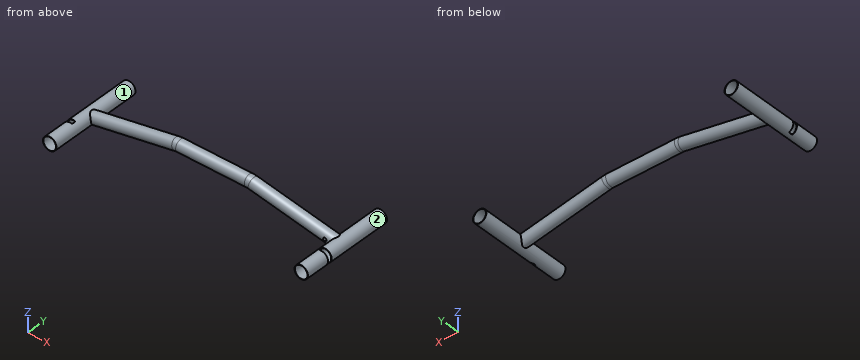
```python
from build123d import *

# Parameters (mm, degrees)
SKETCH2_R               = 11.1
SKETCH2_R_2             = 10.3
SKETCH3_R               = 12.7
SKETCH3_R_2             = 11.9
BOSS_EXTRUDE1_DEPTH     = 88
SKETCH4_R               = 11.9
CUT_EXTRUDE1_DEPTH      = 310.344523999
SKETCH5_R               = 10.7
CUT_EXTRUDE2_DEPTH      = 88
CUT_EXTRUDE3_DEPTH      = 20
CUT_EXTRUDE4_REACH      = 271.188
CUT_EXTRUDE4_END_RADIUS = 11.1
SKETCH8_R               = 3


with BuildPart() as part:
    # Sweep1: sweep along a path in Sketch1
    with BuildLine(Plane(origin=(0, 0, 0), x_dir=(1, 0, 0), z_dir=(0, 1, 0))) as sweep1_path:
        Line((232, 30), (72.22502534, 0.657923176))
        ThreePointArc((72.22502534, 0.657923176), (68.627459651, 0.164820366), (65, 0))
        Line((65, 0), (-65, 0))
        ThreePointArc((-65, 0), (-68.627459651, 0.164820366), (-72.22502534, 0.657923176))
        Line((-72.22502534, 0.657923176), (-232, 30))
    # Sketch2 → Sweep1 (sweep)
    with BuildSketch(Plane(origin=(232, 0, -30), x_dir=(-0.18062563349676417, 0, -0.9835519206040384), z_dir=(0.9835519206040384, 0, -0.18062563349676417))):
        Circle(SKETCH2_R)
        Circle(SKETCH2_R_2, mode=Mode.SUBTRACT)
    sweep(path=sweep1_path.line)

    # Sketch3 → Boss-Extrude1 (add, symmetric)
    with BuildSketch(Plane(origin=(0, 0, 0), x_dir=(1, 0, 0), z_dir=(0, 1, 0))):
        with Locations(Location((237.901311524, 31.083753801, 0), (0, 0, 270))):
            Circle(SKETCH3_R)
        with Locations(Location((237.901311524, 31.083753801, 0), (0, 0, 270))):
            Circle(SKETCH3_R_2, mode=Mode.SUBTRACT)
    boss_extrude1 = extrude(amount=BOSS_EXTRUDE1_DEPTH, both=True)

    # Sketch4 → Cut-Extrude1 (cut, through all)
    with BuildSketch(Plane.XZ.offset(88)):
        with Locations(Location((237.901311524, -31.083753801, 0), (0, 0, 90))):
            Circle(SKETCH4_R)
    cut_extrude1 = extrude(amount=-CUT_EXTRUDE1_DEPTH, mode=Mode.SUBTRACT)

    # Sketch5 → Cut-Extrude2 (cut)
    with BuildSketch(Plane(origin=(232, 0, -30), x_dir=(-0.18062563349676417, 0, -0.9835519206040384), z_dir=(0.9835519206040384, 0, -0.18062563349676417))):
        with Locations((-0.014888445, 0)):
            Circle(SKETCH5_R)
    cut_extrude2 = extrude(amount=-CUT_EXTRUDE2_DEPTH, mode=Mode.SUBTRACT)

    # Sketch7 → Cut-Extrude3 (cut, symmetric)
    with BuildSketch(Plane(origin=(237.901311524, 88, -31.083753801), x_dir=(-0.9420937659324533, 0, -0.3353495731191677), z_dir=(0.33534957311916763, 0, -0.9420937659324532))):
        with BuildLine():
            Line((-2.5, -123.230571249), (-12.7, -123.230571249))
            Line((-12.7, -123.230571249), (-12.7, -131.230571249))
            Line((-12.7, -131.230571249), (-2.5, -131.230571249))
            ThreePointArc((-2.5, -131.230571249), (-0.732233047, -130.498338202), (0, -128.730571249))
            Line((0, -128.730571249), (0, -125.730571249))
            ThreePointArc((0, -125.730571249), (-0.732233047, -123.962804296), (-2.5, -123.230571249))
        make_face()
    cut_extrude3 = extrude(amount=CUT_EXTRUDE3_DEPTH, both=True, mode=Mode.SUBTRACT)

    # Mirror1: Boss-Extrude1, Cut-Extrude1, Cut-Extrude2, Cut-Extrude3 across plane
    add(boss_extrude1.mirror(Plane(origin=(0, 0, 0), x_dir=(0, 0, 1), z_dir=(1, 0, 0))))
    add(cut_extrude1.mirror(Plane(origin=(0, 0, 0), x_dir=(0, 0, 1), z_dir=(1, 0, 0))), mode=Mode.SUBTRACT)
    add(cut_extrude2.mirror(Plane(origin=(0, 0, 0), x_dir=(0, 0, 1), z_dir=(1, 0, 0))), mode=Mode.SUBTRACT)
    add(cut_extrude3.mirror(Plane(origin=(0, 0, 0), x_dir=(0, 0, 1), z_dir=(1, 0, 0))), mode=Mode.SUBTRACT)

    # Cut-Extrude4: up to this cylinder (the profile starts inside it)
    cut_extrude4_end = Plane(origin=(216.872155496, 0, -27.221827908), z_dir=(0.9835519206040384, 0, -0.1806256334967642)) * Cylinder(CUT_EXTRUDE4_END_RADIUS, 565.576, mode=Mode.PRIVATE)
    # Sketch8 → Cut-Extrude4 (cut, up to the surface)
    with BuildSketch(Plane(origin=(0, 0, 0), x_dir=(1, 0, 0), z_dir=(0, 1, 0)), mode=Mode.PRIVATE) as cut_extrude4_sk1:
        with Locations(Location((216.987516382, 26.593661315, 0), (0, 0, 270))):
            Circle(SKETCH8_R)
    cut_extrude4_tool1 = extrude(cut_extrude4_sk1.sketch, amount=-CUT_EXTRUDE4_REACH, mode=Mode.PRIVATE) & cut_extrude4_end
    add(cut_extrude4_tool1.solids().sort_by_distance((216.987516, 0, -26.593661))[0], mode=Mode.SUBTRACT)


solid = part.part
```
Read the model definition and answer for the solid it produces. Units are mm, in the model's axes. Face numbers are marked on the shaded views. Coordinates: 2 decimals unless noted, no trailing zeros. Loops run counter-clockwise (first coordinate to the right, second up) from the corner with the lowest first, then second, coordinate; pieces in that order, holes last. Notation, with made-up numbers: (15, 37) -> (21, 37) arc R14 ccw to (21, 57) -> close; hole circle Ø9 at (30.5, -25). An arc over 180 degrees is marked (long way). Return JSON: item names as keys, results as strings.
Item 1: Find section B-B (y = -22.5). Determine the outline of the cut face in (x, z).
Answers:
{"outline": "circle Ø25.4 at (-237.9, -31.08); circle Ø25.4 at (237.9, -31.08); hole circle Ø23.8 at (-237.9, -31.08); hole circle Ø23.8 at (237.9, -31.08)"}
Item 2: Find section A-A (x = -36.5). Determine the outline of the cut face in (y, z).
Answers:
{"outline": "circle Ø22.2 at (0, 0); hole circle Ø20.6 at (0, 0)"}
Item 3: For a pull along X with two mould halves and no side action, classify the marked faces 1 and 2 as +X half, -X half, draft (parallel to the pull), parting line (faces both ways), or undercut.
Answers:
{"face 1": "undercut", "face 2": "undercut"}
Item 4: Flat-ended cylindrical pins translate along their axes: P1, Ø1, axis at x = 170, z = -9.5, coming from the +Y side; P2, Ø11.5, axis at x = -240.5, z = -27.5, coming from the -Y side; P3, Ø6, axis at x = -45, z = -9, coming from the -Y side; P4, Ø6, axis at x = -125.5, z = -18.5, coming from the -Y side. Find the tip coordinate at first contact, or state that the pin passes through.
Answers:
{"P1": "stops at y = 7.18", "P2": "passes through", "P3": "stops at y = -9.34", "P4": "stops at y = -9.95"}
Item 5: Find the intervals of material crossed by probe 1 along X at (y, z) = (16, -30.5); probe 2 along X at (y, z) = (22, -29.5); probe 3 along Y at (x, z) = (22, 0), in increasing order.
Answers:
{"probe 1": "x = -250.59 to -249.79, -226.02 to -225.21, 225.21 to 226.02, 249.79 to 250.59", "probe 2": "x = -250.5 to -249.7, -226.11 to -225.3, 225.3 to 226.11, 249.7 to 250.5", "probe 3": "y = -11.1 to -10.3, 10.3 to 11.1"}
